```python
from build123d import *

# Parameters (mm, degrees)
SKETCH1_R           = 9.5
BOSS_EXTRUDE1_DEPTH = 25
SKETCH2_R           = 4
CUT_EXTRUDE1_DEPTH  = 12.5
SKETCH3_R           = 2.5
CUT_EXTRUDE2_DEPTH  = 12.5
SKETCH4_R           = 1.25
CUT_EXTRUDE3_DEPTH  = 12.5


with BuildPart() as part:
    # Sketch1 → Boss-Extrude1 (new body)
    with BuildSketch(Plane(origin=(0, 0, 0), x_dir=(1, 0, 0), z_dir=(0, 1, 0))):
        with Locations(Location((0, 0, 0), (0, 0, 270))):
            Circle(SKETCH1_R)
    extrude(amount=BOSS_EXTRUDE1_DEPTH)

    # Sketch2 → Cut-Extrude1 (cut)
    with BuildSketch(Plane(origin=(0, 25, 0), x_dir=(1, 0, 0), z_dir=(0, 1, 0))):
        with Locations(Location((0, 0, 0), (0, 0, 270))):
            Circle(SKETCH2_R)
    extrude(amount=-CUT_EXTRUDE1_DEPTH, mode=Mode.SUBTRACT)

    # Sketch3 → Cut-Extrude2 (cut)
    with BuildSketch(Plane.XZ):
        with Locations(Location((0, 0, 0), (0, 0, 270))):
            Circle(SKETCH3_R)
    extrude(amount=-CUT_EXTRUDE2_DEPTH, mode=Mode.SUBTRACT)

    # Sketch4 → Cut-Extrude3 (cut)
    with BuildSketch(Plane.XY):
        with Locations(Location((0, 4, 0), (0, 0, 90))):
            Circle(SKETCH4_R)
        with Locations((0, 21)):
            Circle(SKETCH4_R)
    extrude(amount=-CUT_EXTRUDE3_DEPTH, mode=Mode.SUBTRACT)


solid = part.part
```
Source: CAD feature listing. Evaluate the final solid. Frame: model axes, mm. A direction names the side the tool comes from. Round coordinates to 2 decimals unless told otherwise and drop trailing zeros. Loops run counter-clockwise (first coordinate to the right, second up) from the corner with the lowest first, then second, coordinate; pieces in that order, holes last. Notation, with made-up numbers: M 40,-35.75 L 53,-35.75 A23 cw 53,-13.75 Z; hole C -21.5,77.5 d2. An arc over 180 degrees is marked long. Put each result on its own line as item: value.
(1) Section D-D, the plane x = -2. Return loops of the section in (y, z).
Solutions:
outline: M 0,-9.29 L 25,-9.29 L 25,-3.46 L 12.5,-3.46 L 12.5,-1.5 L 0,-1.5 Z; M 0,1.5 L 12.5,1.5 L 12.5,3.46 L 25,3.46 L 25,9.29 L 0,9.29 Z
(2) Section C-C, the plane y = 11. Return loops of the section in (x, z).
Solutions:
outline: C 0,0 d19; hole C 0,0 d5
(3) Ray query, line 1 (Z direction, x = 0, y = 17.75); line 2 (Z direction, x = 0, y = 21.75). Return the intervals inside material, ascending. Write a range as [from, to].
Solutions:
line 1: [-9.5, -4], [4, 9.5]
line 2: [4, 9.5]
(4) Access query for faces 4 (the face through (-0.38, 5.19, -5.78)), 5 (the face through (0.1, 6.2, 2.5)), 6 (the face through (2, 12.5, 2)). Directions: +Z, -Z, +X, -X, +Y, -Y. A direction counts if a zero-diameter tool reaches every point of the face in a straight line with its end or side. Return the directions, or none.
Solutions:
face 4: -Z
face 5: +Y, -Y
face 6: +Y
(5) Section A-A, the plane x = 0. Return loops of the section in (y, z).
Solutions:
outline: M 0,-9.5 L 2.75,-9.5 L 2.75,-2.5 L 0,-2.5 Z; M 0,2.5 L 12.5,2.5 L 12.5,4 L 25,4 L 25,9.5 L 0,9.5 Z; M 5.25,-9.5 L 19.75,-9.5 L 19.75,-4 L 12.5,-4 L 12.5,-2.5 L 5.25,-2.5 Z; M 22.25,-9.5 L 25,-9.5 L 25,-4 L 22.25,-4 Z
(6) Pull-direction query (X, two-part tool) for faces 1 (the face through (-3.639, 12.325, 8.776)), 2 (the face through (-1.532, 18.838, 3.695)), 3 (the face through (-4, 25, 2)); classes: released by +X, released by -X, zero draft, split by the parting line, or undercut.
Solutions:
face 1: split by the parting line
face 2: undercut
face 3: zero draft
(7) Section B-B, the plane z = 0. Return loops of the section in (x, y).
Solutions:
outline: M -9.5,0 L -2.5,0 L -2.5,12.5 L -4,12.5 L -4,25 L -9.5,25 Z; M 2.5,0 L 9.5,0 L 9.5,25 L 4,25 L 4,12.5 L 2.5,12.5 Z
(8) First-contact query: pin 1 (1 mm diameter, centred on x = 4, y = 11.5, fed in from -Z); pin 2 (2 mm diameter, centred on x = -1.5, y = 8, fed in from +Z); pin 3 (6 mm diameter, centred on y = 14.5, z = -7, fed in from +X). Flat tips, straight axial feed; report the tip coordinate or a pass-through.
Solutions:
pin 1: z = -8.83
pin 2: z = 9.49
pin 3: x = 8.62
